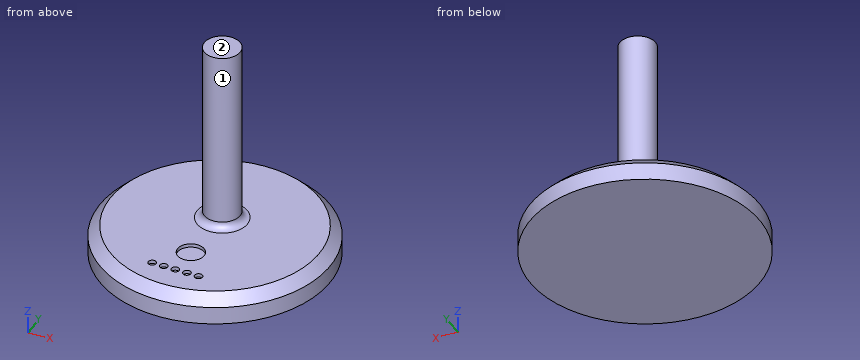
from build123d import *

# Parameters (mm, degrees)
SKETCH034_R     = 160
PAD021_DEPTH    = 40
SKETCH035_R     = 25
PAD022_DEPTH    = 260
FILLET004_R     = 10
SKETCH036_R     = 18.5
SKETCH036_R_2   = 5.5
POCKET004_DEPTH = 5
SKETCH037_R     = 17.5
SKETCH037_R_2   = 5
PAD023_DEPTH    = 10
FILLET005_R     = 1
PAD024_DEPTH    = 5
FILLET006_R     = 0.5
FILLET007_R     = 1.5
FILLET008_R     = 0.5
CHAMFER001_SIZE = 15
SKETCH055_R     = 5
POCKET007_DEPTH = 10
SKETCH056_R     = 17.5
POCKET008_DEPTH = 15


with BuildPart() as part:
    # Sketch034 (on Face1 of CopyPad021) → Pad021 (new body)
    with BuildSketch(Plane(origin=(0, 0, -559.544271), x_dir=(1, 0, 0), z_dir=(0, 0, -1))):
        with Locations((0, -82.297836)):
            Circle(SKETCH034_R)
    extrude(amount=PAD021_DEPTH)

    # Sketch035 (on Face2 of Pad021) → Pad022 (join)
    with BuildSketch(Plane.XY.offset(-559.544271)):
        with Locations((0, 102.297836)):
            Circle(SKETCH035_R)
    extrude(amount=PAD022_DEPTH)

    # Fillet004
    fillet004_edges = [part.edges().sort_by_distance(p)[0] for p in [
        (-25, 102.297836, -559.544271),
    ]]
    fillet(fillet004_edges, radius=FILLET004_R)

    # Sketch036 (on Face1 of Fillet004) → Pocket004 (cut)
    with BuildSketch(Plane.XY.offset(-559.544271)):
        with Locations((0, 15.789559)):
            Circle(SKETCH036_R)
        with Locations((-32.775259, -26.969265)):
            Circle(SKETCH036_R_2)
        with Locations((-16.38763, -26.969265)):
            Circle(SKETCH036_R_2)
        with Locations((0, -26.969265)):
            Circle(SKETCH036_R_2)
        with Locations((16.38763, -26.969265)):
            Circle(SKETCH036_R_2)
        with Locations((32.775259, -26.969265)):
            Circle(SKETCH036_R_2)
    extrude(amount=-POCKET004_DEPTH, mode=Mode.SUBTRACT)

    # Sketch037 (on Face14 of Pocket004) → Pad023 (join)
    with BuildSketch(Plane.XY.offset(-564.544271)):
        with Locations((0, 15.789559)):
            Circle(SKETCH037_R)
        with Locations((-32.775259, -26.969265)):
            Circle(SKETCH037_R_2)
        with Locations((-16.38763, -26.969265)):
            Circle(SKETCH037_R_2)
        with Locations((0, -26.969265)):
            Circle(SKETCH037_R_2)
        with Locations((16.38763, -26.969265)):
            Circle(SKETCH037_R_2)
        with Locations((32.775259, -26.969265)):
            Circle(SKETCH037_R_2)
    extrude(amount=PAD023_DEPTH)

    # Fillet005
    fillet005_edges = [part.edges().sort_by_distance(p)[0] for p in [
        (-5, -26.969265, -554.544271),
        (11.38763, -26.969265, -554.544271),
        (27.775259, -26.969265, -554.544271),
        (-21.38763, -26.969265, -554.544271),
        (-37.775259, -26.969265, -554.544271),
    ]]
    fillet(fillet005_edges, radius=FILLET005_R)

    # Sketch038 (on Face29 of Fillet005) → Pad024 (join)
    with BuildSketch(Plane.XY.offset(-554.544271)):
        with BuildLine():
            ThreePointArc((3.946719, 28.587051), (0, 32.53377), (-3.946719, 28.587051))
            Line((-3.946719, 28.587051), (-3.946719, 2.992067))
            ThreePointArc((-3.946719, 2.992067), (0, -0.954652), (3.946719, 2.992067))
            Line((3.946719, 28.587051), (3.946719, 2.992067))
        make_face()
    extrude(amount=PAD024_DEPTH)

    # Fillet006
    fillet006_edges = [part.edges().sort_by_distance(p)[0] for p in [
        (-3.946719, 15.789559, -554.544271),
    ]]
    fillet(fillet006_edges, radius=FILLET006_R)

    # Fillet007
    fillet007_edges = [part.edges().sort_by_distance(p)[0] for p in [
        (-3.946719, 15.789559, -549.544271),
    ]]
    fillet(fillet007_edges, radius=FILLET007_R)

    # Fillet008
    fillet008_edges = [part.edges().sort_by_distance(p)[0] for p in [
        (-17.5, 15.789559, -554.544271),
    ]]
    fillet(fillet008_edges, radius=FILLET008_R)

    # Chamfer001
    chamfer001_edges = [part.edges().sort_by_distance(p)[0] for p in [
        (-160, 82.297836, -559.544271),
    ]]
    chamfer(chamfer001_edges, length=CHAMFER001_SIZE)

    # Sketch055 (on Face36 of Chamfer001) → Pocket007 (cut)
    with BuildSketch(Plane.XY.offset(-554.544271)):
        with Locations((-32.775259, -26.969265)):
            Circle(SKETCH055_R)
        with Locations((-16.38763, -26.969265)):
            Circle(SKETCH055_R)
        with Locations((0, -26.969265)):
            Circle(SKETCH055_R)
        with Locations((16.38763, -26.969265)):
            Circle(SKETCH055_R)
        with Locations((32.775259, -26.969265)):
            Circle(SKETCH055_R)
    extrude(amount=-POCKET007_DEPTH, mode=Mode.SUBTRACT)

    # Sketch056 (on Face30 of Pocket007) → Pocket008 (cut)
    with BuildSketch(Plane.XY.offset(-549.544271)):
        with Locations((0, 15.789559)):
            Circle(SKETCH056_R)
    extrude(amount=-POCKET008_DEPTH, mode=Mode.SUBTRACT)


with BuildPart() as part_1:
    # Clone002 placement: moved
    add(part.part.moved(Location((0, 0, 599.54))))


solid = part_1.part
Can you work these out from the model? Positions are in its coordinate system, mm. Face numbers are marked on the shaded views. A direction names the side the tool comes from. Round coordinates to 2 decimals unless told otherwise and drop trailing zeros. Write each loop counter-clockwise with the first axis right and the second up, starting at its lowest first coordinate (ties: lowest second). Pieces come first, ordered by that corner, then holes. Notation, with made-up numbers: (12.5, -39.5) -> (21.5, -39.5) arc R12 ccw to (21.5, -21.5) -> close; hole circle Ø5 at (-35.75, -17.5). An arc over 180 degrees is marked (long way). One line per question, with ' | ' between items. Start each with the question number.
1) On a 3-axis mill with a long thin cutter (end or side, diameter ignored), from which of +Z, -Z, +X, -X, +Y, -Y can I reach the whole of each face in a straight line? I mean the marked faces 1 and 2. Say none if no direction works.
2) Suppose I cut it at A-A on x = 0. Write out the boundary of the cut face in (y, z), then the cut area to 3 significant figures.
3) I'm going to push flat-ended pins straight in: P1, Ø5.5, axis at x = 1.5, y = -24.5, coming from the +Z side; P2, Ø10, axis at x = -16.39, y = -26.97, coming from the +Z side; P3, Ø8, axis at x = -8, z = 129, coming from the +Y side. Where does each tip first touch, or does it pass through?
4) Suppose I cut it at B-B on z = 248.5. Write out the boundary of the cut face in (x, y), then the cut area to 3 significant figures.
5) I need wall thicknesses on line 1 (Y direction, x = 0, z = 36.75); line 2 (X direction, y = 85.5, z = 141); line 3 (X direction, y = 119, z = 231). Which ranges of each line are inside material? Lowest first, please. Write a range as [from, to].
Return value:
1) face 1: +Z | face 2: +Z, +X, -X, +Y, -Y
2) outline: (-77.7, 0) -> (242.3, 0) -> (242.3, 25) -> (227.3, 40) -> (137.3, 40) arc R10 cw to (127.3, 50) -> (127.3, 300) -> (77.3, 300) -> (77.3, 50) arc R10 cw to (67.3, 40) -> (34.29, 40) -> (34.29, 35) -> (-2.71, 35) -> (-2.71, 40) -> (-21.47, 40) -> (-21.47, 35) -> (-32.47, 35) -> (-32.47, 40) -> (-62.7, 40) -> (-77.7, 25) -> close | area: 25,400 mm2
3) P1: stops at z = 40 | P2: stops at z = 35 | P3: stops at y = 126.98
4) outline: circle Ø50 at (0, 102.3) | area: 1,960 mm2
5) line 1: y = [-65.95, -32.47], [-21.47, -2.71], [34.29, 230.54] | line 2: x = [-18.52, 18.52] | line 3: x = [-18.6, 18.6]
